Model file for the job. Use its own axes, mm. A direction names the side the tool comes from. Coordinates: 2 decimals unless noted, no trailing zeros. Loops run counter-clockwise (first coordinate to the right, second up) from the corner with the lowest first, then second, coordinate; pieces in that order, holes last.
from build123d import *

# Parameters (mm, degrees)
F1_R     = 12.7
F4_R     = 6.35
F5_DEPTH = 75


with BuildPart() as f2:
    # F2: sweep along a path in F0
    with BuildLine(Plane.XZ) as f2_path:
        Line((0, 0), (0, 76.2))
        ThreePointArc((0, 76.2), (14.8789755157, 112.1210244843), (50.8, 127))
        Line((50.8, 127), (127, 127))
    # F1 (on Top) → F2 (sweep)
    with BuildSketch(Plane.XY):
        Circle(F1_R)
    sweep(path=f2_path.line)

    # F4 (on offset) → F5 (join)
    with BuildSketch(Plane.YZ.offset(-25.4)):
        with Locations((0, 127)):
            Circle(F4_R)
    extrude(amount=F5_DEPTH)


solid = f2.part
Q1. Slice it at B-B (x = 86). List the corners of the cut face in (y, z), and give its area (3 significant figures).
Answers:
outline: circle Ø25.4 at (0, 127)
area: 507 mm2
Q2. Drill centre lines: line 1 (X direction, y = -0.75, z = 10.5); line 2 (Z direction, x = 72, y = 1); line 3 (Y direction, x = 103, z = 126). Where is each one in solid material? Low to high.
Answers:
line 1: x = -12.68 to 12.68
line 2: z = 114.34 to 139.66
line 3: y = -12.66 to 12.66
Q3. Slice it at D-D (y = 9). List the corners of the cut face in (x, z), and give its area (3 significant figures).
Answers:
outline: (-8.96, 0) - (8.96, 0) - (8.96, 76.2) arc R41.84 cw to (50.8, 118.04) - (127, 118.04) - (127, 135.96) - (50.8, 135.96) arc R59.76 ccw to (-8.96, 76.2) - close
area: 4,160 mm2
Q4. Flat gauge pins, fed straight in: P1, Ø8, axis at x = 26, z = 104.5, coming from the -Y side; P2, Ø5, axis at x = 78.5, z = 115, coming from the -Y side; P3, Ø10, axis at x = 88, z = 122.5, coming from the +Y side; P4, Ø8, axis at y = 2, z = 85.5, coming from the -X side. Where does each tip first touch, or does it go through?
Answers:
P1: stops at y = -8.79
P2: stops at y = -8.43
P3: stops at y = 12.7
P4: stops at x = -12.44
Q5. Slice it at A-A (y = -2.5). List the corners of the cut face in (x, z).
Answers:
outline: (-25.4, 121.16) - (6.31, 121.16) arc R63.25 ccw to (-12.45, 76.2) - (-12.45, 0) - (12.45, 0) - (12.45, 76.2) arc R38.35 cw to (50.8, 114.55) - (127, 114.55) - (127, 139.45) - (50.8, 139.45) arc R63.25 ccw to (22.64, 132.84) - (-25.4, 132.84) - close
Q6. Slice it at C-C (z = 58). List the corners of the cut face in (x, y).
Answers:
outline: circle Ø25.4 at (0, 0)
Q7. Which spindle directions (+Z, -Z, +X, -X, +Y, -Y) get a long thin tool onto all of the face, cutting with end or side? Do faces 1 (the cylindrical face through (-2.75, -12.4, 38.63)), 2 (the cylindrical face through (-6.9, -0.8, 133.3)), 3 (the cylindrical face through (89.433, 0.558, 139.688)). Say none if no direction does.
Answers:
face 1: -Z
face 2: -X
face 3: +X
